Can you work these out from the model? Positions are in its coordinate system, mm. Face numbers are marked on the shaded views. Give positions to 0.01 mm unless a question says otherwise; leave off trailing zeros. Order: outer loops, then holes, each group sorted by start corner. A loop starts at its lowest first (then second) coordinate and runs counter-clockwise, first axis right, second up.
```python
from build123d import *

# Parameters (mm, degrees)
SKETCH_1_W          = 105
SKETCH_1_H          = 120
EXTRUDE_1_DEPTH     = 4
SKETCH_4_W          = 25
SKETCH_4_H          = 4
CUT_EXTRUDE_1_DEPTH = 155
CUT_EXTRUDE_3_DEPTH = 155
SHELL_1_T           = -1


with BuildPart() as part:
    # 스케치1 → 보스-돌출1 (new body)
    with BuildSketch(Plane(origin=(0, 0, 0), x_dir=(1, 0, 0), z_dir=(0, 1, 0))):
        Rectangle(SKETCH_1_W, SKETCH_1_H)
    extrude(amount=EXTRUDE_1_DEPTH)

    # 스케치4 → 컷-돌출1 (cut)
    with BuildSketch(Plane.XY.offset(60)):
        with Locations((40, 2)):
            Rectangle(SKETCH_4_W, SKETCH_4_H)
    extrude(amount=-CUT_EXTRUDE_1_DEPTH, mode=Mode.SUBTRACT)

    # 스케치6 → 컷-돌출3 (cut)
    with BuildSketch(Plane.XY.offset(60)):
        Polygon((-52.5, 4), (-52.5, 1), (27.5, 4), align=None)
    extrude(amount=-CUT_EXTRUDE_3_DEPTH, mode=Mode.SUBTRACT)

    # 쉘1
    shell_1_openings = [part.faces().sort_by_distance(p)[0] for p in [
        (-12.5, 0, 0),
    ]]
    offset(amount=SHELL_1_T, openings=shell_1_openings, kind=Kind.INTERSECTION)


solid = part.part
```
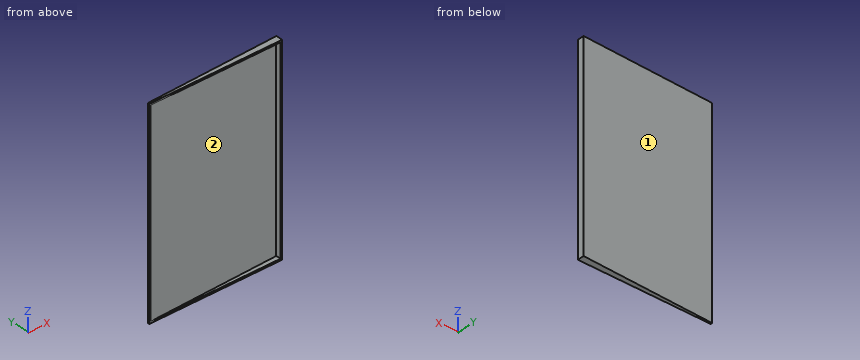
1) We'd pull the mould along X, two halves only. Please class the marked faces 1 and 2: +X half, -X half, draft (parallel to the pull), parting line (faces both ways), or undercut.
2) Suppose I cut it at B-B (y = 1.65). Please give me the cut outline in (x, z).
3) Suppose I cut it at C-C (x = -9.5). Please give me the cut outline in (y, z), and give its area (3 significant figures).
4) I'm going to push flat-ended pins straight in: pin 1 Ø4 at (x, z) = (-40.5, -15) entering from +Y (3 decimals); pin 2 Ø2 at (x, z) = (19, 12.5) entering from +Y; pin 3 Ø10 at (x, z) = (5, -10) entering from -Y. Where does each tip first touch, or does it pass through?
5) If I drill on line 1 (Z direction, x = 7, y = 2.05); line 2 (Y direction, x = -43, z = 42.5); line 3 (Y direction, x = -26, z = -1.5), over which ranges is the centre line in solid material (lowest first)?
Results:
1. face 1: -X half
1. face 2: undercut
2. outline: (-35.17, -60) - (27.5, -60) - (27.5, 60) - (-35.17, 60) - close; hole (-8.48, -59) - (26.5, -59) - (26.5, 59) - (-8.48, 59) - close
3. outline: (0, -60) - (2.61, -60) - (2.61, 60) - (0, 60) - (0, 59) - (1.61, 59) - (1.61, -59) - (0, -59) - close
3. area: 123 mm2
4. pin 1: stops at y = 1.525
4. pin 2: stops at y = 3.72
4. pin 3: stops at y = 1.97
5. line 1: z = -60 to -59, 59 to 60
5. line 2: y = 0.36 to 1.36
5. line 3: y = 0.99 to 1.99
